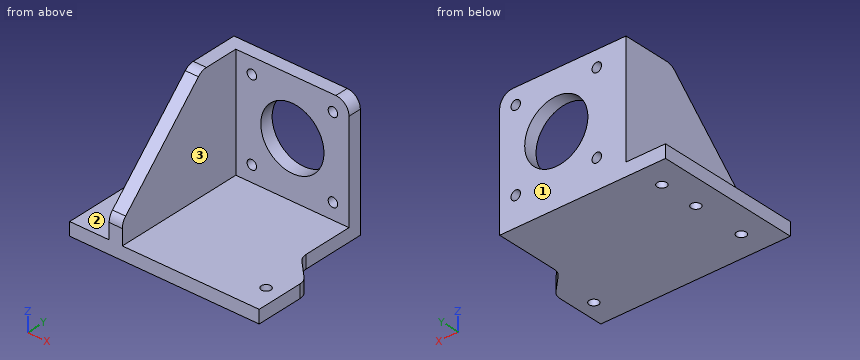
```python
from build123d import *

# Parameters (mm, degrees)
F1_DEPTH = 5
F2_R     = 1.8
F3_DEPTH = 25
F5_DEPTH = 43
F7_DEPTH = 25
F8_R     = 12
F8_R_2   = 1.8
F9_DEPTH = 25
F10_R    = 5


with BuildPart() as f1:
    # F0 (on Top) → F1 (new body)
    with BuildSketch(Plane.XY):
        Polygon((-36, 27.5), (-36, -27.5), (36, -27.5), (36, -7.5), (27, 1.5), (27, 27.5), align=None)
    extrude(amount=F1_DEPTH)

    # F2 (on face) → F3 (cut)
    with BuildSketch(Plane.XY.offset(5)):
        with Locations((-26, 17.5)):
            Circle(F2_R)
        with Locations((-26, 2.5)):
            Circle(F2_R)
        with Locations((-26, -17.5)):
            Circle(F2_R)
        with Locations((30, -17.5)):
            Circle(F2_R)
    extrude(amount=-F3_DEPTH, mode=Mode.SUBTRACT)

    # F4 (on face) → F5 (join)
    with BuildSketch(Plane.XY.offset(5)):
        Polygon((-16, 22.5), (27, 22.5), (27, 27.5), (-21, 27.5), (-21, -27.5), (-16, -27.5), align=None)
    extrude(amount=F5_DEPTH)

    # F6 (on face) → F7 (cut)
    with BuildSketch(Plane.YZ.offset(-16)):
        Polygon((-27.5, 13), (7.5, 48), (-27.5, 48), align=None)
    extrude(amount=-F7_DEPTH, mode=Mode.SUBTRACT)

    # F8 (on face) → F9 (cut)
    with BuildSketch(Plane.XZ.offset(-22.5)):
        with Locations((5.5, 26.5)):
            Circle(F8_R)
        with Locations((-9.9, 41.9)):
            Circle(F8_R_2)
        with Locations((-9.9, 11.1)):
            Circle(F8_R_2)
        with Locations((20.9, 41.9)):
            Circle(F8_R_2)
        with Locations((20.9, 11.1)):
            Circle(F8_R_2)
    extrude(amount=-F9_DEPTH, mode=Mode.SUBTRACT)

    # F10
    f10_edges = [f1.edges().sort_by_distance(p)[0] for p in [
        (-18.5, 7.5, 48),
        (-18.5, -27.5, 13),
        (27, 25, 48),
        (36, -7.5, 2.5),
        (27, 1.5, 2.5),
    ]]
    fillet(f10_edges, radius=F10_R)


solid = f1.part
```
Part model, mm, in its own coordinate system. Face numbers are marked on the shaded views. A direction names the side the tool comes from. Give positions to 0.01 mm unless a question says otherwise; leave off trailing zeros. Order: outer loops, then holes, each group sorted by start corner. A loop starts at its lowest first (then second) coordinate and runs counter-clockwise, first axis right, second up. Notation, with made-up numbers: M 81.5,-40 L 88.5,-40 A14 ccw 88.5,-14 Z; hole C 7.25,7.25 d7. An arc over 180 degrees is marked long. Use a Markdown table: item, result. Add a question column.
(1) Probe line 1 along X through (y, z) = (26, 11); line 2 along Y through (x, z) = (-26, 3); line 3 along X through (y, z) = (7, 15.5). List the from-to ranges inside material, lowest first. Write a range as [from, to].
(2) Saw through at A-A, the plane x = -9.9. Give the cut face in (y, z).
(3) Drop flat-ended pins along their axis: P1, Ø4, axis at y = 6.5, z = 42.5, coming from the -X side; P2, Ø1.5, axis at x = 24.5, y = 10, coming from the +Z side; P3, Ø7, axis at y = 18, z = 27.5, coming from the +X side; P4, Ø4, axis at x = -9.9, z = 41.9, coming from the +Y side. Give the stop position or say it passes through.
(4) Saw through at D-D, the plane y = 2.5. Give the cut face in (x, z).
(5) 3-axis set-ups, long thin cutter, end or side, ignore diameter. For the marked faces 1, 2 and 3: which of +Z, -Z, +X, -X, +Y, -Y reach the whole face in a straight line?
(6) Saw through at C-C, the plane x = -19. Give the cut face in (y, z).
(7) Saw through at B-B, the plane z = 26.5. Give the cut face in (x, y), and give its area (4 significant figures).
Answer key:
| question | item | result |
|---|---|---|
| 1 | line 1 | [-21, -11.7], [-8.1, 19.1], [22.7, 27] |
| 1 | line 2 | [-27.5, -19.3], [-15.7, 0.7], [4.3, 15.7], [19.3, 27.5] |
| 1 | line 3 | [-21, -16] |
| 2 | outline | M -27.5,0 L 27.5,0 L 27.5,9.3 L 22.5,9.3 L 22.5,5 L -27.5,5 Z; M 22.5,12.9 L 27.5,12.9 L 27.5,40.1 L 22.5,40.1 Z; M 22.5,43.7 L 27.5,43.7 L 27.5,48 L 22.5,48 Z |
| 3 | P1 | x = -21 |
| 3 | P2 | z = 5 |
| 3 | P3 | x = -16 |
| 3 | P4 | y = 27.5 |
| 4 | outline | M -36,0 L -27.8,0 L -27.8,5 L -36,5 Z; M -24.2,0 L 27.12,0 L 27.12,5 L -16,5 L -16,43 L -21,43 L -21,5 L -24.2,5 Z |
| 5 | face 1 | +Z, -Z, +X, -X, +Y |
| 5 | face 2 | +Z, -X, +Y, -Y |
| 5 | face 3 | +Z, +X, -Y |
| 6 | outline | M -27.5,0 L 27.5,0 L 27.5,48 L 9.57,48 A5 ccw 6.04,46.54 L -26.04,14.46 A5 ccw -27.5,10.93 Z |
| 7 | outline | M -21,-14 L -16,-14 L -16,22.5 L -6.5,22.5 L -6.5,27.5 L -21,27.5 Z; M 17.5,22.5 L 27,22.5 L 27,27.5 L 17.5,27.5 Z |
| 7 | area | 302.5 mm^2 |
